Work out the finished part from the listing and answer in its coordinate system (mm). A direction names the side the tool comes from. Coordinates: 2 decimals unless noted, no trailing zeros. Order: outer loops, then holes, each group sorted by start corner. A loop starts at its lowest first (then second) coordinate and runs counter-clockwise, first axis right, second up. Notation, with made-up numbers: M -22.75,-22 L 22.25,-22 A17 ccw 22.25,-16 Z; hole C 0,25.5 d4. An arc over 180 degrees is marked long. Write item = value, one per line. Start each with the question number.
Q1. Determine the mould class of faces 3 (the flat face through (0, 8, 2)), 4 (the flat face through (12, 0, 2)), 5 (the flat face through (25, 12.7, 2)) for opening direction X: released by +X, released by -X, zero draft, split by the parting line, or undercut.
Q2. Straight lines are drawn through the part: line 1 along X through (y, z) = (13, 1.4); line 2 along Y through (x, z) = (18, 0.75); line 3 along X through (y, z) = (4.25, 2.5). For each, find the intervals that lie inside material, in ascending order.
Q3. Find section D-D on y = 5. Give the vertices of the cut face in (x, z) (3 decimals).
Q4. A tool of negligible diameter and unlimited length cuts with its end or side. For faces 1 (the flat face through (25, 10, 3.175)), 2 (the flat face through (12.7, 14, 2)), from which of +Z, -Z, +X, -X, +Y, -Y can it reach the whole face along a straight path? Write none if from no direction.
Q5. Find section B-B on z = 2.4. Give the vertices of the cut face in (x, y) (3 decimals), and give its area (3 significant figures).
Q6. Find section C-C on x = 30.5. Give the vertices of the cut face in (y, z) (3 decimals), and give its area (3 significant figures).
Q7. Find section A-A on y = 13.25. Give the vertices of the cut face in (x, z) (3 decimals).
```python
from build123d import *

# Parameters (mm, degrees)
SKETCH1_W       = 50.8
SKETCH1_H       = 12.7
EXTRUDE1_DEPTH  = 3.175
SKETCH3_W       = 12.7
SKETCH3_H       = 3.175
EXTRUDE3_DEPTH  = 3.175
LPATTERN1_COUNT = 2
LPATTERN1_PITCH = 38.1
EXTRUDE4_DEPTH  = 4.175


with BuildPart() as part:
    # Sketch1 → Extrude1 (new body)
    with BuildSketch(Plane.XY):
        with Locations((25.4, 6.35)):
            Rectangle(SKETCH1_W, SKETCH1_H)
    extrude(amount=EXTRUDE1_DEPTH)

    # Sketch3 → Extrude3 (add)
    with BuildSketch(Plane(origin=(0, 12.7, 0), x_dir=(1, 0, 0), z_dir=(0, 1, 0))):
        with Locations((6.35, -1.5875)):
            Rectangle(SKETCH3_W, SKETCH3_H)
    extrude3 = extrude(amount=EXTRUDE3_DEPTH)

    # LPattern1: Extrude3 ×2
    with Locations(*[(i * LPATTERN1_PITCH, 0, 0) for i in range(1, LPATTERN1_COUNT)]):
        add(extrude3)

    # Sketch4 → Extrude4 (cut, through all)
    with BuildSketch(Plane.XY.offset(3.175)):
        with BuildLine():
            Line((27.391652548, 6.144928853), (27.441911715, 0.016746365))
            ThreePointArc((27.441911715, 0.016746365), (25.416746365, -2.041911715), (23.358088285, -0.016746365))
            Line((23.358088285, -0.016746365), (23.307829118, 6.111436122))
            ThreePointArc((23.307829118, 6.111436122), (25.332994468, 8.170094203), (27.391652548, 6.144928853))
        make_face()
    extrude(amount=-EXTRUDE4_DEPTH, mode=Mode.SUBTRACT)


solid = part.part
```
Findings below:
q1.face_3 = released by -X
q1.face_4 = zero draft
q1.face_5 = undercut
q2.line_1 = 0 to 12.7, 38.1 to 50.8
q2.line_2 = 0 to 12.7
q2.line_3 = 0 to 23.32, 27.41 to 50.8
q3.outline = M 0,0 L 23.317,0 L 23.317,3.175 L 0,3.175 Z; M 27.401,0 L 50.8,0 L 50.8,3.175 L 27.401,3.175 Z
q4.face_1 = +Z, +X, -X, +Y, -Y
q4.face_2 = +Z, -Z, +Y
q5.outline = M 0,0 L 23.358,0 L 23.308,6.111 A2.042 cw 27.392,6.145 L 27.442,0.017 A2.042 cw 27.442,0 L 50.8,0 L 50.8,15.875 L 38.1,15.875 L 38.1,12.7 L 12.7,12.7 L 12.7,15.875 L 0,15.875 Z
q5.area = 694 mm^2
q6.outline = M 0,0 L 12.7,0 L 12.7,3.175 L 0,3.175 Z
q6.area = 40.3 mm^2
q7.outline = M 0,0 L 12.7,0 L 12.7,3.175 L 0,3.175 Z; M 38.1,0 L 50.8,0 L 50.8,3.175 L 38.1,3.175 Z
